Could you check a few things on this model? Use its own coordinates, in mm. A direction names the side the tool comes from. Give positions to 0.01 mm unless a question says otherwise; leave off trailing zeros. Write each loop counter-clockwise with the first axis right and the second up, starting at its lowest first coordinate (ties: lowest second). Pieces come first, ordered by that corner, then holes. Notation, with made-up numbers: (87, -17.75) - (125, -17.75) arc R20 ccw to (125, 13.25) - close; hole circle Ø5 at (84, 44). An arc over 180 degrees is marked (long way). Use one line per item in the form item = value.
```python
from build123d import *

# Parameters (mm, degrees)
IZIM1_R                     = 14
Y_KSEKLIK_EKSTR_ZYON1_DEPTH = 5
PAH1_SIZE                   = 5
PAH1_SIZE_2                 = 0.881634904
BO_ALTMA1_T                 = -2
IZIM2_R                     = 4.5
KES_EKSTR_ZYON1_DEPTH       = 3
KES_EKSTR_ZYON2_REACH       = 22.421
IZIM3_R                     = 1.5


with BuildPart() as part:
    # Çizim1 → Yükseklik-Ekstrüzyon1 (new body)
    with BuildSketch(Plane(origin=(0, 0, 0), x_dir=(1, 0, 0), z_dir=(0, 1, 0))):
        with Locations(Location((0, 0, 0), (0, 0, 270))):
            Circle(IZIM1_R)
    extrude(amount=Y_KSEKLIK_EKSTR_ZYON1_DEPTH)

    # Pah1
    # the kernel refuses this chamfer: 5, 0.881634904 mm, written as the material it takes off along each edge
    with BuildSketch(Plane(origin=(0, 0, 0), x_dir=(0, 0, 1), z_dir=(-1, 0, 0))) as pah1_piece_1:
        Polygon((14, PAH1_SIZE), (14 - PAH1_SIZE_2, 0), (14, 0), align=None)
    revolve(axis=Axis((0, 0, 0), (0, 1, 0)), mode=Mode.SUBTRACT)

    # İç Boşaltma1
    bo_altma1_openings = [part.faces().sort_by_distance(p)[0] for p in [
        (0, 5, 0),
    ]]
    offset(amount=BO_ALTMA1_T, openings=bo_altma1_openings, kind=Kind.INTERSECTION)

    # Çizim2 → Kes-Ekstrüzyon1 (cut)
    with BuildSketch(Plane.XZ):
        with BuildLine():
            ThreePointArc((-7.5, 11.821590418), (0, 8.435968695), (7.5, 11.821590418))
            ThreePointArc((7.5, 11.821590418), (0, 14), (-7.5, 11.821590418))
        make_face()
        with Locations(Location((0, 0, 0), (0, 0, 270))):
            Circle(IZIM2_R)
        with BuildLine():
            ThreePointArc((11.821590418, -7.5), (14, 0), (11.821590418, 7.5))
            ThreePointArc((11.821590418, 7.5), (8.435968695, 0), (11.821590418, -7.5))
        make_face()
        with BuildLine():
            ThreePointArc((-7.5, -11.821590418), (0, -14), (7.5, -11.821590418))
            ThreePointArc((7.5, -11.821590418), (0, -8.435968695), (-7.5, -11.821590418))
        make_face()
        with BuildLine():
            ThreePointArc((-11.821590418, 7.5), (-14, 0), (-11.821590418, -7.5))
            ThreePointArc((-11.821590418, -7.5), (-8.435968695, 0), (-11.821590418, 7.5))
        make_face()
    extrude(amount=-KES_EKSTR_ZYON1_DEPTH, mode=Mode.SUBTRACT)

    # Çizim3 → Kes-Ekstrüzyon2 (cut, up to next)
    with BuildSketch(Plane.XZ, mode=Mode.PRIVATE) as kes_ekstr_zyon2_sk1:
        with Locations(Location((-5.656854249, 5.656854249, 0), (0, 0, 270))):
            Circle(IZIM3_R)
    kes_ekstr_zyon2_tool1 = extrude(kes_ekstr_zyon2_sk1.sketch, amount=-KES_EKSTR_ZYON2_REACH, mode=Mode.PRIVATE) & part.part
    # Çizim3 → Kes-Ekstrüzyon2 (cut, up to next)
    with BuildSketch(Plane.XZ, mode=Mode.PRIVATE) as kes_ekstr_zyon2_sk2:
        with Locations(Location((6.717514421, 6.717514421, 0), (0, 0, 270))):
            Circle(IZIM3_R)
    kes_ekstr_zyon2_tool2 = extrude(kes_ekstr_zyon2_sk2.sketch, amount=-KES_EKSTR_ZYON2_REACH, mode=Mode.PRIVATE) & part.part
    # Çizim3 → Kes-Ekstrüzyon2 (cut, up to next)
    with BuildSketch(Plane.XZ, mode=Mode.PRIVATE) as kes_ekstr_zyon2_sk3:
        with Locations(Location((5.656854249, -5.656854249, 0), (0, 0, 270))):
            Circle(IZIM3_R)
    kes_ekstr_zyon2_tool3 = extrude(kes_ekstr_zyon2_sk3.sketch, amount=-KES_EKSTR_ZYON2_REACH, mode=Mode.PRIVATE) & part.part
    # Çizim3 → Kes-Ekstrüzyon2 (cut, up to next)
    with BuildSketch(Plane.XZ, mode=Mode.PRIVATE) as kes_ekstr_zyon2_sk4:
        with Locations(Location((-6.717514421, -6.717514421, 0), (0, 0, 270))):
            Circle(IZIM3_R)
    kes_ekstr_zyon2_tool4 = extrude(kes_ekstr_zyon2_sk4.sketch, amount=-KES_EKSTR_ZYON2_REACH, mode=Mode.PRIVATE) & part.part
    add(kes_ekstr_zyon2_tool1.solids().sort_by_distance((-5.656854, 0, 5.656854))[0], mode=Mode.SUBTRACT)
    add(kes_ekstr_zyon2_tool2.solids().sort_by_distance((6.717514, 0, 6.717514))[0], mode=Mode.SUBTRACT)
    add(kes_ekstr_zyon2_tool3.solids().sort_by_distance((5.656854, 0, -5.656854))[0], mode=Mode.SUBTRACT)
    add(kes_ekstr_zyon2_tool4.solids().sort_by_distance((-6.717514, 0, -6.717514))[0], mode=Mode.SUBTRACT)


solid = part.part
```
1. For pin 1 (2.5 mm diameter, centred on x = -6.72, z = -6.72, fed in from +Y); pin 2 (3 mm diameter, centred on y = 1.5, z = 10.5, fed in from -X); pin 3 (1 mm diameter, centred on x = 8, z = 2, fed in from +Y); pin 4 (1 mm diameter, centred on x = -2.5, z = 11, fed in from -Y), each with a flat end and sliding along its axis, tell me the tip position at first contact or that it passes through.
Response values:
pin_1 = through
pin_2 = -9.95
pin_3 = 2
pin_4 = 3
2. Which directions (+Z, -Z, +X, -X, +Y, -Y) give clear straight access to the entire face, cutting with the end or side of a thin tool? Please do faces 4 (the face through (0, 2, -5)), 5 (the face through (-12, 3, 0)), 6 (the face through (0.114, 1.146, -8.437)), 7 (the face through (-0.114, 1.146, 8.437)).
Response values:
face_4 = +Y
face_5 = -X, -Y
face_6 = -Z, -Y
face_7 = +Z, -Y
3. If I drill on line 1 (X direction, y = 1.65, z = 0); line 2 (Y direction, x = -6, z = -1.25); line 3 (X direction, y = 3.5, z = -8.5), over which ranges is the centre line in solid material (lowest first)? Write a range as from..to.
Response values:
line_1 = -8.44..-4.5, 4.5..8.44
line_2 = 0..2
line_3 = -10.79..-8.05, 8.05..10.79
4. Imagine slicing it at A-A, the plane x = 0. List the corners of the cut face in (y, z) for me, and give its area (3 significant figures).
Response values:
outline = (0, -8.44) - (2, -8.44) - (2, -4.5) - (0, -4.5) - close; (0, 4.5) - (2, 4.5) - (2, 8.44) - (0, 8.44) - close; (3, -13.65) - (5, -14) - (5, -11.97) - (3, -11.62) - close; (3, 11.62) - (5, 11.97) - (5, 14) - (3, 13.65) - close
area = 23.9 mm²
5. Imagine slicing it at D-D, the plane y = 4. List the corners of the cut face in (x, z) for me.
Response values:
outline = circle Ø27.65 at (0, 0); hole circle Ø23.59 at (0, 0)
6. Imagine slicing it at C-C, the plane y = 1.3. List the corners of the cut face in (x, z) for me, and give its area (3 significant figures).
Response values:
outline = (-11.34, -7.04) arc R13.35 ccw to (-7.04, -11.34) arc R10 cw to (7.04, -11.34) arc R13.35 ccw to (11.34, -7.04) arc R10 cw to (11.34, 7.04) arc R13.35 ccw to (7.04, 11.34) arc R10 cw to (-7.04, 11.34) arc R13.35 ccw to (-11.34, 7.04) arc R10 cw to start; hole circle Ø3 at (-6.72, -6.72); hole circle Ø3 at (-5.66, 5.66); hole circle Ø9 at (0, 0); hole circle Ø3 at (5.66, -5.66); hole circle Ø3 at (6.72, 6.72)
area = 278 mm²
7. Imagine slicing it at B-B, the plane z = 0. List the corners of the cut face in (x, y) for me.
Response values:
outline = (-14, 5) - (-13.65, 3) - (-11.62, 3) - (-11.97, 5) - close; (-8.44, 0) - (-4.5, 0) - (-4.5, 2) - (-8.44, 2) - close; (4.5, 0) - (8.44, 0) - (8.44, 2) - (4.5, 2) - close; (11.62, 3) - (13.65, 3) - (14, 5) - (11.97, 5) - close
8. If we mould it in two halves opening along X, with no side actions, what happens to faces 1 (the face through (1.352, 0.986, -4.292)), 2 (the face through (12, 3, 0)), 3 (the face through (8.437, 1.146, 0.114))? For each: pulls with the +X half, pulls with the -X half, needs draft (parallel to the pull), parting line crosses it, or undercut.
Response values:
face_1 = undercut
face_2 = needs draft
face_3 = pulls with the +X half
